Here's how the part is built. I have some questions about the finished solid (model axes, mm). Face numbers are marked on the shaded views. A direction names the side the tool comes from. Give positions to 0.01 mm unless a question says otherwise; leave off trailing zeros. Loops run counter-clockwise (first coordinate to the right, second up) from the corner with the lowest first, then second, coordinate; pieces in that order, holes last.
Q1. If we section it at C-C (x = -18): Please give me the cut outline in (y, z) (3 decimals).
Q2. We'd pull the mould along X, two halves only. Please class the marked faces 5, 6, 7 and 8: +X half, -X half, draft (parallel to the pull), parting line (faces both ways), or undercut.
Q3. I need wall thicknesses on line 1 (X direction, y = 9, z = 30); line 2 (Z direction, x = -27.5, y = 9.5); line 3 (Z direction, x = 2, y = 13) (3 decimals). Which ranges of each line are inside material? Lowest first, please.
Q4. For the marked faces 1, 2, 3 and 4, which set-ups out of +Z, -Z, +X, -X, +Y, -Y let a thin tool reach every point of the face, with its end or its side?
Q5. Will these pins go through, and if not, where does the flat tip stop? P1, Ø6, axis at x = -29, z = 9.5, coming from the +Y side; P2, Ø5, axis at x = 8, y = 7.5, coming from the +Z side; P3, Ø11, axis at y = 11, z = -15.5, coming from the +X side.
Q6. If we section it at B-B (y = 15.5): Please give me the cut outline in (x, z), plus the area to 3 significant figures.
Q7. If we section it at D-D (z = -29.5): Please give me the cut outline in (x, y), plus the area to 3 significant figures.
Q8. If we section it at A-A (y = 8.5): Please give me the cut outline in (x, z) (3 decimals).
from build123d import *

# Parameters (mm, degrees)
SKETCH1_W            = 100
SKETCH1_H            = 100
BOSS_EXTRUDE1_DEPTH  = 4
SKETCH2_W            = 91.5
SKETCH2_H            = 91.5
SKETCH2_W_2          = 83.5
SKETCH2_H_2          = 83.5
BOSS_EXTRUDE2_DEPTH  = 35
SKETCH3_W            = 4
SKETCH3_H            = 4
CUT_EXTRUDE1_DEPTH   = 4
SKETCH4_W            = 26
SKETCH4_H            = 2.75
SKETCH4_W_2          = 3
SKETCH4_H_2          = 44.42
BOSS_EXTRUDE3_DEPTH  = 10
SKETCH5_W            = 50
SKETCH5_H            = 1.375
CUT_EXTRUDE2_DEPTH   = 79.89866919
SKETCH7_W            = 4
SKETCH7_H            = 4
BOSS_EXTRUDE5_DEPTH  = 4
SKETCH8_W            = 87.495245403
SKETCH8_H            = 87.5
CUT_EXTRUDE6_DEPTH   = 25
SKETCH10_W           = 87.495245403
SKETCH10_H           = 87.5
SKETCH10_W_2         = 83.5
SKETCH10_H_2         = 83.5
CUT_EXTRUDE8_DEPTH   = 10
SKETCH11_OUTSIDE_W   = 131.34
SKETCH11_OUTSIDE_H   = 131.34
SKETCH11_OUTSIDE_W_2 = 96
SKETCH11_OUTSIDE_H_2 = 96
CUT_EXTRUDE9_DEPTH   = 32
SKETCH12_W           = 96
SKETCH12_H           = 2
CUT_EXTRUDE10_DEPTH  = 115.197197864


with BuildPart() as part:
    # Sketch1 → Boss-Extrude1 (new body)
    with BuildSketch(Plane(origin=(0, 0, 0), x_dir=(1, 0, 0), z_dir=(0, 1, 0))):
        Rectangle(SKETCH1_W, SKETCH1_H)
    extrude(amount=BOSS_EXTRUDE1_DEPTH)

    # Sketch2 → Boss-Extrude2 (add)
    with BuildSketch(Plane(origin=(0, 4, 0), x_dir=(1, 0, 0), z_dir=(0, 1, 0))):
        Rectangle(SKETCH2_W, SKETCH2_H)
        Rectangle(SKETCH2_W_2, SKETCH2_H_2, mode=Mode.SUBTRACT)
    extrude(amount=BOSS_EXTRUDE2_DEPTH)

    # Sketch3 → Cut-Extrude1 (cut)
    with BuildSketch(Plane(origin=(0, 0, -45.75), x_dir=(-1, 0, 0), z_dir=(0, 0, -1))):
        with Locations((0, 6)):
            Rectangle(SKETCH3_W, SKETCH3_H)
    extrude(amount=-CUT_EXTRUDE1_DEPTH, mode=Mode.SUBTRACT)

    # Sketch4 → Boss-Extrude3 (add)
    with BuildSketch(Plane(origin=(0, 4, 0), x_dir=(1, 0, 0), z_dir=(0, 1, 0))):
        Polygon((-28, 22.21), (-25, 22.21), (-25, 39), (-13, 39), (-13, 41.75), (-28, 41.75), align=None)
        Polygon((25, 39), (25, 22.21), (28, 22.21), (28, 41.75), (13, 41.75), (13, 39), align=None)
        Polygon((25, -39), (13, -39), (13, -41.75), (28, -41.75), (28, -22.21), (25, -22.21), align=None)
        Polygon((-13, -39), (-25, -39), (-25, -22.21), (-28, -22.21), (-28, -41.75), (-13, -41.75), align=None)
        with Locations((0, -40.375)):
            Rectangle(SKETCH4_W, SKETCH4_H)
        with Locations((-26.5, 0)):
            Rectangle(SKETCH4_W_2, SKETCH4_H_2)
        with Locations((0, 40.375)):
            Rectangle(SKETCH4_W, SKETCH4_H)
        with Locations((26.5, 0)):
            Rectangle(SKETCH4_W_2, SKETCH4_H_2)
    extrude(amount=BOSS_EXTRUDE3_DEPTH)

    # Sketch5 → Cut-Extrude2 (cut, through all)
    with BuildSketch(Plane(origin=(0, 4, 0), x_dir=(1, 0, 0), z_dir=(0, 1, 0))):
        with Locations((0, 39.6875)):
            Rectangle(SKETCH5_W, SKETCH5_H)
    extrude(amount=CUT_EXTRUDE2_DEPTH, mode=Mode.SUBTRACT)

    # Sketch7 → Boss-Extrude5 (add)
    with BuildSketch(Plane(origin=(0, 0, -45.75), x_dir=(-1, 0, 0), z_dir=(0, 0, -1))):
        with Locations((0, 6)):
            Rectangle(SKETCH7_W, SKETCH7_H)
    extrude(amount=-BOSS_EXTRUDE5_DEPTH)

    # Sketch8 → Cut-Extrude6 (cut)
    with BuildSketch(Plane(origin=(0, 39, 0), x_dir=(1, 0, 0), z_dir=(0, 1, 0))):
        with Locations((0.002377298, 0)):
            Rectangle(SKETCH8_W, SKETCH8_H)
    extrude(amount=-CUT_EXTRUDE6_DEPTH, mode=Mode.SUBTRACT)

    # Sketch10 → Cut-Extrude8 (cut)
    with BuildSketch(Plane(origin=(0, 14, 0), x_dir=(1, 0, 0), z_dir=(0, 1, 0))):
        with Locations((0.002377298, 0)):
            Rectangle(SKETCH10_W, SKETCH10_H)
        Rectangle(SKETCH10_W_2, SKETCH10_H_2, mode=Mode.SUBTRACT)
    extrude(amount=-CUT_EXTRUDE8_DEPTH, mode=Mode.SUBTRACT)

    # Sketch11 outside → Cut-Extrude9 (cut)
    with BuildSketch(Plane(origin=(0, 4, 0), x_dir=(1, 0, 0), z_dir=(0, 1, 0))):
        Rectangle(SKETCH11_OUTSIDE_W, SKETCH11_OUTSIDE_H)
        Rectangle(SKETCH11_OUTSIDE_W_2, SKETCH11_OUTSIDE_H_2, mode=Mode.SUBTRACT)
    extrude(amount=-CUT_EXTRUDE9_DEPTH, mode=Mode.SUBTRACT)

    # Sketch12 → Cut-Extrude10 (cut, through all)
    with BuildSketch(Plane(origin=(0, 0, -48), x_dir=(-1, 0, 0), z_dir=(0, 0, -1))):
        with Locations((0, 1)):
            Rectangle(SKETCH12_W, SKETCH12_H)
    extrude(amount=-CUT_EXTRUDE10_DEPTH, mode=Mode.SUBTRACT)


solid = part.part
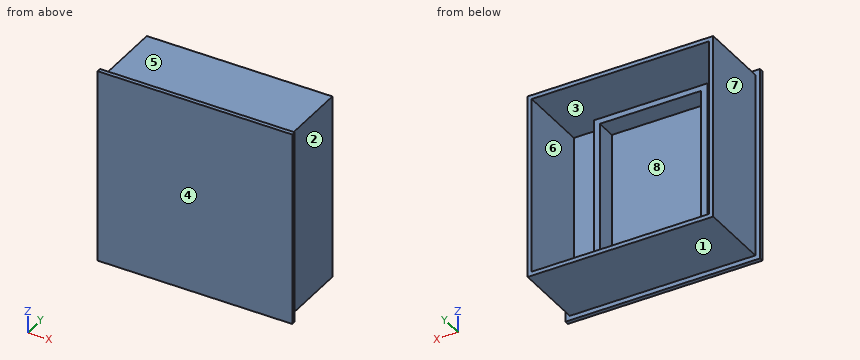
Check sheet entries:
1. outline: (2, -48) - (4, -48) - (4, -45.75) - (39, -45.75) - (39, -43.75) - (4, -43.75) - (4, -41.75) - (14, -41.75) - (14, -40.375) - (4, -40.375) - (4, 39) - (14, 39) - (14, 41.75) - (4, 41.75) - (4, 43.75) - (39, 43.75) - (39, 45.75) - (4, 45.75) - (4, 48) - (2, 48) - close
2. face 5: draft
2. face 6: undercut
2. face 7: -X half
2. face 8: undercut
3. line 1: x = -45.75 to -43.75, -28 to -25, 25 to 28, 43.75 to 45.75
3. line 2: z = -45.75 to -43.75, -41.75 to 41.75, 43.75 to 45.75
3. line 3: z = -45.75 to -43.75, -41.75 to -40.375, 39 to 41.75, 43.75 to 45.75
4. face 1: -Z, +X, -X, +Y
4. face 2: +Z, -Z, +X, +Y
4. face 3: +Y
4. face 4: +Z, -Z, +X, -X, -Y
5. P1: stops at y = 14
5. P2: stops at z = 45.75
5. P3: stops at x = 45.75
6. outline: (-45.75, -45.75) - (45.75, -45.75) - (45.75, 45.75) - (-45.75, 45.75) - close; hole (-43.75, -43.75) - (43.75, -43.75) - (43.75, 43.75) - (-43.75, 43.75) - close
6. area: 716 mm2
7. outline: (-48, 2) - (48, 2) - (48, 4) - (45.75, 4) - (45.75, 39) - (43.75, 39) - (43.75, 4) - (28, 4) - (28, 14) - (25, 14) - (25, 4) - (-25, 4) - (-25, 14) - (-28, 14) - (-28, 4) - (-43.75, 4) - (-43.75, 39) - (-45.75, 39) - (-45.75, 4) - (-48, 4) - close
7. area: 392 mm2
8. outline: (-45.75, -45.75) - (45.75, -45.75) - (45.75, 45.75) - (-45.75, 45.75) - close; (-28, -41.75) - (28, -41.75) - (28, 41.75) - (-28, 41.75) - close; hole (-43.745, -43.75) - (43.75, -43.75) - (43.75, 43.75) - (-43.745, 43.75) - close; hole (-25, -40.375) - (25, -40.375) - (25, 39) - (-25, 39) - close
